Design review of the part built by this model. Coordinates are the model's own, in mm. A direction names the side the tool comes from. Give positions to 0.01 mm unless a question says otherwise; leave off trailing zeros. Loops run counter-clockwise (first coordinate to the right, second up) from the corner with the lowest first, then second, coordinate; pieces in that order, holes last. Notation, with made-up numbers: (54.25, 49.5) -> (66.25, 49.5) arc R28 ccw to (66.25, 70.5) -> close; hole circle Ø10 at (70, 53). An arc over 180 degrees is marked (long way). Use a Markdown table: item, result. Add a question column.
1. Add section C-C (x = 1.75). State the section outline as (y, z) points (3 decimals), and give its area (3 significant figures).
2. Draft analysis for pull direction Z (two halves, no side actions). For faces 1 (the flat face through (-4.575, -3, 12)), 2 (the cylindrical face through (10.158, -3.153, -18.282)), 3 (the cylindrical face through (10.164, -3.219, -0.358)), state which applies: pulls with the +Z half, pulls with the -Z half, needs draft (parallel to the pull), parting line crosses it, or undercut.
3. For pin 1 Ø3.5 at (y, z) = (-4.5, -2) entering from +X; pin 2 Ø1 at (y, z) = (-3.5, 4) entering from +X; pin 3 Ø1.5 at (y, z) = (-1.5, -6) entering from -X, all flat-tipped, find the tip position at first contact; note any pin that passes through.
4. Add section B-B (z = 10.5). State the section outline as (x, y) points, and give its area (3 significant figures).
5. For faces 4 (the flat face through (-2, -6.35, 3)), 5 (the flat face through (-1, -3, -3.175)), 6 (the flat face through (5, -3, 3.175)), list the 3-axis set-ups (+Z, -Z, +X, -X, +Y, -Y) from which the entire face can be reached by the end or side of a thin tool; tool diameter is ignored.
6. To check wall thickness, follow line 1 (Z direction, x = -1.5, y = -3.75) (3 decimals); line 2 (Z direction, x = -7.5, y = -2.5) (1 decimal); line 3 (X direction, y = -3.5, z = 15.5). State the ranges of each line that lie inside material, in increasing order.
```python
from build123d import *

# Parameters (mm, degrees)
F0_W     = 6.35
F0_H     = 14.2875
F1_DEPTH = 6.35
F2_D     = 2.38125
F2_DEPTH = 6.35
F2_TIP   = 0.7153996745
F3_R     = 1.5875
F4_R     = 3.175


with BuildPart() as f1:
    # F0 (on Front) → F1 (new body)
    with BuildSketch(Plane.XZ):
        with Locations((-7.7499226887, 10.31875)):
            Rectangle(F0_W, F0_H)
        Polygon((14.4750773113, -3.175), (14.4750773113, 3.175), (-4.5749226887, 3.175), (-10.9249226887, 3.175), (-10.9249226887, -3.175), (8.1250773113, -3.175), align=None)
        with BuildLine():
            ThreePointArc((14.8093424829, -29.9953674142), (13.0855162795, -16.6045849499), (14.4750773113, -3.175))
            Line((14.4750773113, -3.175), (8.1250773113, -3.175))
            ThreePointArc((8.1250773113, -3.175), (9.821316188, -16.995379057), (14.8093424829, -29.9953674142))
        make_face()
    extrude(amount=F1_DEPTH)

    # F2
    with Locations(Plane(origin=(0, 0, 0), x_dir=(1, 0, 0), z_dir=(0, 1, 0))):
        with Locations((11.3000773113, 0)):
            Hole(F2_D / 2, depth=F2_DEPTH)
            with Locations((0, 0, -(F2_DEPTH + F2_TIP / 2))):  # 118° drill point
                Cone(0, F2_D / 2, F2_TIP, mode=Mode.SUBTRACT)

    # F3
    f3_edges = [f1.edges().sort_by_distance(p)[0] for p in [
        (13.085516, -6.35, -16.604585),
        (9.821316, -6.35, -16.995379),
        (13.085516, 0, -16.604585),
        (9.821316, 0, -16.995379),
    ]]
    fillet(f3_edges, radius=F3_R)

    # F4
    f4_edges = [f1.edges().sort_by_distance(p)[0] for p in [
        (14.475077, -3.175, 3.175),
        (-10.924923, -3.175, -3.175),
        (-4.574923, -3.175, 3.175),
        (8.125077, -3.175, -3.175),
    ]]
    fillet(f4_edges, radius=F4_R)


solid = f1.part
```
Taken from the geometry:
| question | item | result |
|---|---|---|
| 1 | outline | (-6.35, -3.175) -> (0, -3.175) -> (0, 3.175) -> (-6.35, 3.175) -> close |
| 1 | area | 40.3 mm^2 |
| 2 | face 1 | needs draft |
| 2 | face 2 | pulls with the -Z half |
| 2 | face 3 | undercut |
| 3 | pin 1 | stops at x = 14.48 |
| 3 | pin 2 | stops at x = -2.8 |
| 3 | pin 3 | stops at x = 8.01 |
| 4 | outline | (-10.92, -6.35) -> (-4.57, -6.35) -> (-4.57, 0) -> (-10.92, 0) -> close |
| 4 | area | 40.3 mm^2 |
| 5 | face 4 | +Z, -Z, +X, -X, -Y |
| 5 | face 5 | -Z, -X, +Y, -Y |
| 5 | face 6 | +Z, +X, +Y, -Y |
| 6 | line 1 | z = -3.175 to 3.177 |
| 6 | line 2 | z = -3.2 to 17.5 |
| 6 | line 3 | x = -10.92 to -4.57 |
